Here's how the part is built. I have some questions about the finished solid (model axes, mm). Round coordinates to 2 decimals unless told otherwise and drop trailing zeros. Loops run counter-clockwise (first coordinate to the right, second up) from the corner with the lowest first, then second, coordinate; pieces in that order, holes last. Notation, with made-up numbers: M -33,-23.75 L -19,-23.75 A28 ccw -19,6.25 Z; hole C 15.25,-9 d11. An arc over 180 degrees is marked long. Put each result on its own line as item: value. Start each with the question number.
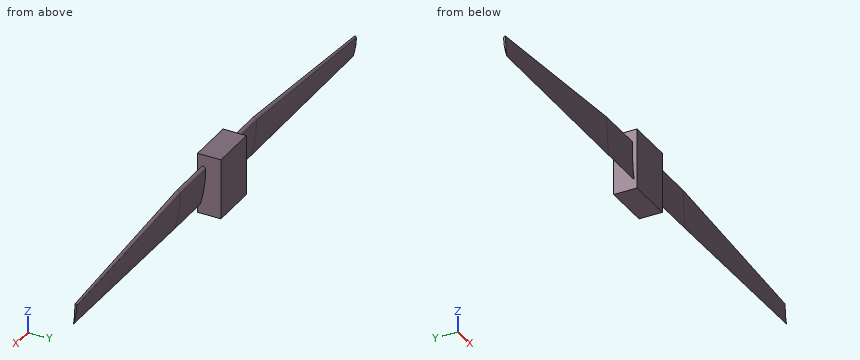
Autodesk Inventor part; units mm, degrees
ref_plane "YZ Plane" through (0, 0, 0) normal (1, 0, 0) x (0, 1, 0)
ref_plane "XZ Plane" through (0, 0, 0) normal (0, 1, 0) x (-1, 0, 0)
ref_plane "XY Plane" through (0, 0, 0) normal (0, 0, 1) x (1, 0, 0)
sketch "Sketch1" plane through (0, 0, 0) normal (0, 1, 0) x (-1, 0, 0)
  line L0 (115.4545, -16.1636) -> (-138.5455, -16.1636)
  line L1 (-138.5455, -16.1636) -> (-138.5455, -346.3636)
  line L2 (-138.5455, -346.3636) -> (115.4545, -346.3636)
  line L3 (115.4545, -346.3636) -> (115.4545, -16.1636)
  point P0 (0, 0)
  dimension "d0" = 254
  dimension "d1" = 330.2
extrude "Extrusion1" add sketch "Sketch1" along normal blind 127
sketch "Sketch2" plane through (138.5455, 0, -16.1636) normal (1, 0, 0) x (0, 0, -1)
  arc A0 (76.2, 44.45) -> (63.5, 25.4) centre (81.0618, 27.4505) ccw
  line L0 (76.2, 44.45) -> (177.2082, 44.45) construction
  line L1 (177.2082, 44.45) -> (279.4, 15.24) construction
  spline S0 degree 2 poles (76.2, 44.45) (177.2082, 44.45) (279.4, 15.24) knots 1 1 1 2 2 2
  line L2 (63.5, 25.4) -> (224.9578, 24.13) construction
  line L3 (224.9578, 24.13) -> (279.4, 15.24) construction
  spline S1 degree 2 poles (63.5, 25.4) (224.9578, 24.13) (279.4, 15.24) knots 1 1 1 2 2 2
  line L4 (0, 0) -> (330.2, 0)
  line L5 (0, 127) -> (330.2, 127)
  line L6 (0, 0) -> (0, 127)
  line L7 (330.2, 0) -> (330.2, 127)
  point P0 (-16.1636, 0)
  dimension "d4" = 25.4
  dimension "d5" = 15.24
  dimension "d6" = 24.13
  dimension "d7" = 82.55
  dimension "d8" = 82.55
  dimension "d9" = 63.5
  dimension "d10" = 76.2
  dimension "d11" = 50.8
  dimension "d12" = 101.0082
  dimension "d13" = 102.1918
extrude "Extrusion2" add sketch "Sketch2" along normal blind 254 and the other way blind 508 contours S0 S1 A0
ref_plane "Work Plane1" through (1408.5455, 0, -16.1636) normal (1, 0, 0) x (0, 0, -1)
sketch "Sketch5" plane through (1408.5455, 0, -16.1636) normal (1, 0, 0) x (0, 0, -1)
  arc A0 (76.2, 44.45) -> (63.5, 25.4) centre (81.0618, 27.4505) ccw
  spline S0 degree 2 poles (154.1033, 24.5678) (240.1651, 22.1028) (269.0908, 16.7605) knots 1 1 1 2 2 2
  spline S1 degree 2 poles (269.0908, 16.7605) (214.934, 33.4644) (161.0849, 34.5831) knots 1 1 1 2 2 2
  arc A1 (161.0849, 34.5831) -> (154.1033, 24.5678) centre (163.4885, 25.4665) ccw
  point P0 (-16.1636, 0)
loft "Loft1" add profiles "Sketch5" section 1 edges at (392.5455, 22.225, -214.3675) (392.5455, 37.1475, -193.6678) (392.5455, 37.2582, -82.5139)
ref_plane "Work Plane3" through (-1385.4545, 0, -16.1636) normal (-1, 0, 0) x (0, 0, 1)
sketch "Sketch7" plane through (-1385.4545, 0, -16.1636) normal (-1, 0, 0) x (0, 0, 1)
  spline S0 degree 2 poles (-269.0908, 16.7605) (-240.1651, 22.1028) (-154.1033, 24.5678) knots 0 0 0 1 1 1
  spline S1 degree 2 poles (-161.0849, 34.5831) (-214.934, 33.4644) (-269.0908, 16.7605) knots 0 0 0 1 1 1
  arc A0 (-154.1033, 24.5678) -> (-161.0849, 34.5831) centre (-163.4885, 25.4665) ccw
  point P0 (16.1636, 0)
loft "Loft2" add profiles "Sketch7" section 2 edges at (-369.4545, 22.225, -214.3675) (-369.4545, 37.2582, -82.5139) (-369.4545, 37.1475, -193.6678)
properties part number "Glider Box"
1) I'm going to push flat-ended pins straight in: P1, Ø1, axis at y = 111.5, z = -147, coming from the +X side; P2, Ø3, axis at x = -378, z = -227.5, coming from the +Y side; P3, Ø6, axis at x = -707, z = -283, coming from the -Y side. Where does each tip first touch, or does it pass through?
2) If I drill on probe 1 along X at (y, z) = (10, -71); probe 2 along Y at (x, z) = (454, -287); probe 3 along Y at (x, z) = (725.5, -198), over which ranges is the centre line in solid material (lowest first)? Write a range as from..to.
3) Suppose I cut it at A-A (y = 94). Write out the boundary of the cut face in (x, z).
Results are:
1. P1: x = 138.55
1. P2: y = 31.76
1. P3: y = 16.69
2. probe 1: -115.45..138.55
2. probe 2: 16.51..17.56
2. probe 3: 23.07..35.79
3. outline: M -115.45,-346.36 L 138.55,-346.36 L 138.55,-16.16 L -115.45,-16.16 Z
